Geometry check sheet. Reference: the model listing, model coordinates, mm. A direction names the side the tool comes from. Give positions to 0.01 mm unless a question says otherwise; leave off trailing zeros. Loops run counter-clockwise (first coordinate to the right, second up) from the corner with the lowest first, then second, coordinate; pieces in that order, holes last. Notation, with made-up numbers: (-19.5, 25) - (8.5, 25) arc R18 ccw to (8.5, 51) - close; hole circle Ø10 at (42.5, 84.5). An arc over 180 degrees is marked (long way). One line per question, with ' | ' between items. Start each with the question number.
from build123d import *

# Parameters (mm, degrees)
SKETCH1_W           = 50
SKETCH1_H           = 16
BOSS_EXTRUDE1_DEPTH = 2
SKETCH2_R           = 1.575
BOSS_EXTRUDE2_DEPTH = 3
SKETCH3_W           = 31
SKETCH3_H           = 12
CUT_EXTRUDE1_DEPTH  = 3
FILLET1_R           = 2
FILLET2_R           = 2
SKETCH4_R           = 2.325
BOSS_EXTRUDE3_DEPTH = 8


with BuildPart() as part:
    # Sketch1 → Boss-Extrude1 (new body)
    with BuildSketch(Plane.XY):
        with Locations((25, 8)):
            Rectangle(SKETCH1_W, SKETCH1_H)
    extrude(amount=BOSS_EXTRUDE1_DEPTH)

    # Sketch2 → Boss-Extrude2 (add)
    with BuildSketch(Plane.XY.offset(2)):
        with Locations(Location((6.675, 8, 0), (0, 0, 180))):
            Circle(SKETCH2_R)
        with Locations(Location((43.675, 8, 0), (0, 0, 180))):
            Circle(SKETCH2_R)
    extrude(amount=BOSS_EXTRUDE2_DEPTH)

    # Sketch3 → Cut-Extrude1 (cut)
    with BuildSketch(Plane.XY.offset(2)):
        with Locations((25, 8)):
            Rectangle(SKETCH3_W, SKETCH3_H)
    extrude(amount=-CUT_EXTRUDE1_DEPTH, mode=Mode.SUBTRACT)

    # Fillet1
    fillet1_edges = [part.edges().sort_by_distance(p)[0] for p in [
        (9.5, 2, 1),
        (9.5, 14, 1),
        (40.5, 14, 1),
        (40.5, 2, 1),
    ]]
    fillet(fillet1_edges, radius=FILLET1_R)

    # Fillet2
    fillet2_edges = [part.edges().sort_by_distance(p)[0] for p in [
        (0, 16, 1),
        (50, 16, 1),
        (50, 0, 1),
        (0, 0, 1),
    ]]
    fillet(fillet2_edges, radius=FILLET2_R)

    # Sketch4 → Boss-Extrude3 (add)
    with BuildSketch(Plane(origin=(0, 0, 0), x_dir=(-1, 0, 0), z_dir=(0, 0, -1))):
        with Locations((-44.643589023, 8)):
            Circle(SKETCH4_R)
        with Locations((-4.643589023, 8)):
            Circle(SKETCH4_R)
    extrude(amount=BOSS_EXTRUDE3_DEPTH)


solid = part.part
(1) Material ranges on line 1 (X direction, y = 6, z = 0.5); line 2 (Y direction, x = 19, z = 0.75); line 3 (Z direction, x = 42, y = 7), recorded low to high.
(2) Section check B-B, the plane y = 8. Record the boundary of the cut face in (x, z).
(3) Section check D-D, the plane y = 12.5. Record the boundary of the cut face in (x, z).
(4) Mould release check, pull along Y, two halves, no side actions. Record for faces 1 (the face through (5, 8, -8)), 2 (the face through (2.426, 8.698, -3.944)), 3 (the face through (25, 0, 1)), 4 (the face through (39.9, 2.57, 0.99)): pulls with the +Y half, pulls with the -Y half, needs draft (parallel to the pull), parting line crosses it, or undercut.
(5) Depth check by flat-ended pin: pin 1 Ø1.5 at (y, z) = (9, -4) entering from +X; pin 2 Ø6 at (x, z) = (5.5, -5.5) entering from -Y (3 decimals); pin 3 Ø5 at (x, y) = (32, 5.5) entering from -Z; pin 4 Ø5 at (x, z) = (8.5, -5.5) entering from +Y. Enter the tip coordinate at first touch or a pass-through.
(6) Section check C-C, the plane z = 3.5. Record the boundary of the cut face in (x, y) (3 decimals).
(7) Section check A-A, the plane x = 24. Record the boundary of the cut face in (y, z), and give its area (3 significant figures).
(8) Tool access check on faces 5 (the face through (45.25, 7.93, 3.48)), 6 (the face through (46.966, 8.102, -3.944)), 7 (the face through (50, 8, 1)), 8 (the face through (39.93, 13.4, 0.99)). Record the directions out of +Z, -Z, +X, -X, +Y, -Y that give a thin tool (end or side, any length) a straight path to the whole face; none if there is none.
Numbers:
1) line 1: 0 to 9.5, 40.5 to 50 | line 2: 0 to 2, 14 to 16 | line 3: 0 to 2
2) outline: (0, 0) - (2.32, 0) - (2.32, -8) - (6.97, -8) - (6.97, 0) - (9.5, 0) - (9.5, 2) - (8.25, 2) - (8.25, 5) - (5.1, 5) - (5.1, 2) - (0, 2) - close; (40.5, 0) - (42.32, 0) - (42.32, -8) - (46.97, -8) - (46.97, 0) - (50, 0) - (50, 2) - (45.25, 2) - (45.25, 5) - (42.1, 5) - (42.1, 2) - (40.5, 2) - close
3) outline: (0, 0) - (9.56, 0) - (9.56, 2) - (0, 2) - close; (40.44, 0) - (50, 0) - (50, 2) - (40.44, 2) - close
4) face 1: needs draft | face 2: parting line crosses it | face 3: pulls with the -Y half | face 4: undercut
5) pin 1: x = 46.96 | pin 2: y = 5.675 | pin 3: through | pin 4: y = 9.89
6) outline: circle Ø3.15 at (6.675, 8); circle Ø3.15 at (43.675, 8)
7) outline: (0, 0) - (2, 0) - (2, 2) - (0, 2) - close; (14, 0) - (16, 0) - (16, 2) - (14, 2) - close | area: 8.00 mm^2
8) face 5: +Z | face 6: -Z | face 7: +Z, -Z, +X, +Y, -Y | face 8: +Z, -Z
